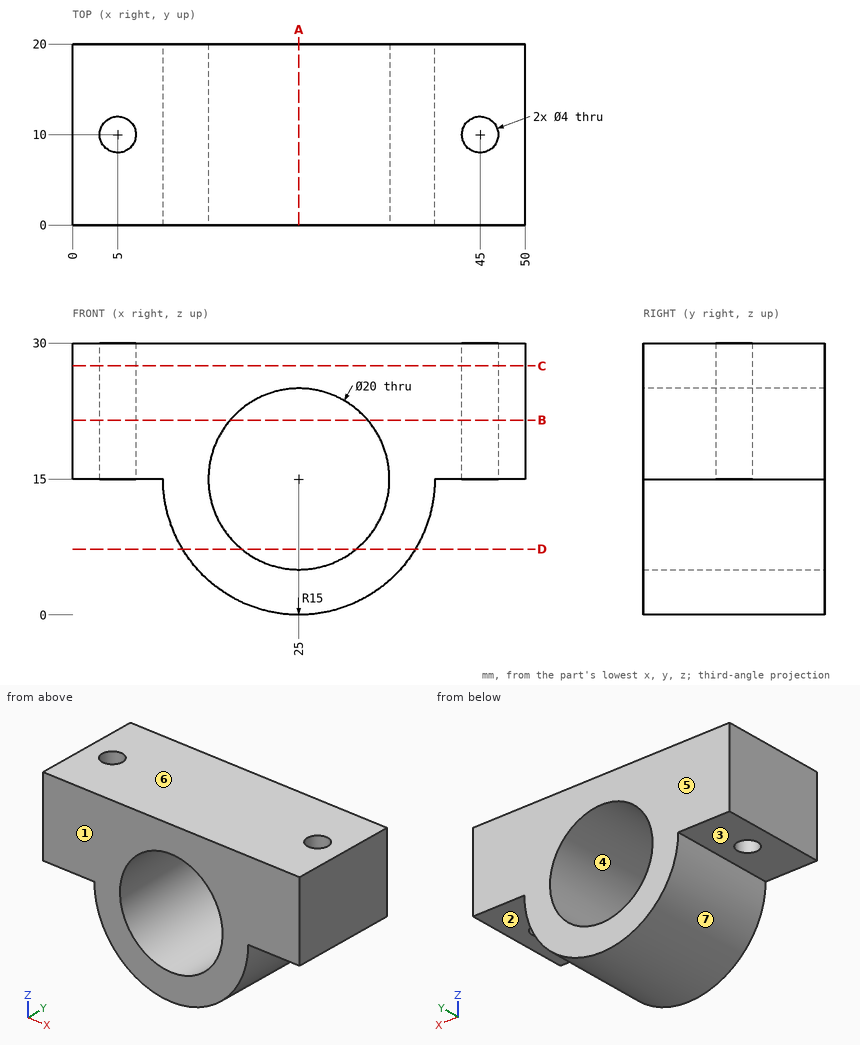
Input: dimensioned drawing with shaded views. Units: mm. Origin: part minimum x, y, z. A direction names the side the tool comes from. Give positions to 0.01 mm unless a question says otherwise; leave off trailing zeros. Order: outer loops, then holes, each group sorted by start corner. A loop starts at its lowest first (then second) coordinate and runs counter-clockwise, first axis right, second up. Notation, with made-up numbers: (22.5, 41.5) -> (33.5, 41.5) arc R19 cw to (33.5, 66.5) -> close; hole circle Ø2 at (-15, 40.25). An arc over 180 degrees is marked (long way). Use a Markdown table: item, result.
1) Section query B-B, the plane z = 21.5. Return the cut outline in (x, y), then the cut area to 3 significant figures.
Answer list:
| item | result |
|---|---|
| outline | (0, 0) -> (17.4, 0) -> (17.4, 20) -> (0, 20) -> close; (32.6, 0) -> (50, 0) -> (50, 20) -> (32.6, 20) -> close; hole circle Ø4 at (5, 10); hole circle Ø4 at (45, 10) |
| area | 671 mm² |
2) Ray query, line 1 along Y through (x, z) = (45, 20); line 2 along Z through (x, y) = (45, 2.5); line 3 along X through (y, z) = (3, 17). Return the intervals inside material, ascending. Write a range as [from, to].
Answer list:
| item | result |
|---|---|
| line 1 | [0, 8], [12, 20] |
| line 2 | [15, 30] |
| line 3 | [0, 15.2], [34.8, 50] |
3) Section query D-D, the plane z = 7.25. Return the cut outline in (x, y).
Answer list:
| item | result |
|---|---|
| outline | (12.16, 0) -> (18.68, 0) -> (18.68, 20) -> (12.16, 20) -> close; (31.32, 0) -> (37.84, 0) -> (37.84, 20) -> (31.32, 20) -> close |
4) Contact query for flat-ended pins moving along their axis: P1, Ø5, axis at x = 45.5, y = 8, coming from the -Z side; P2, Ø12, axis at x = 25.5, z = 17, coming from the -Y side; P3, Ø2, axis at y = 14.5, z = 8, coming from the -X side. Output: stop coordinate, or through.
Answer list:
| item | result |
|---|---|
| P1 | z = 15 |
| P2 | through |
| P3 | x = 11.25 |
5) Section query A-A, the plane x = 25. Return the cut outline in (y, z), then the cut area to 3 significant figures.
Answer list:
| item | result |
|---|---|
| outline | (0, 0) -> (20, 0) -> (20, 5) -> (0, 5) -> close; (0, 25) -> (20, 25) -> (20, 30) -> (0, 30) -> close |
| area | 200 mm² |
6) Reachability of the marked faces 1, 2 and 3 from +Z, -Z, +X, -X, +Y, -Y: full face, straight path, thin tool, end or side. Return the list, or none.
Answer list:
| item | result |
|---|---|
| face 1 | +Z, -Z, +X, -X, -Y |
| face 2 | -Z, +X, +Y, -Y |
| face 3 | -Z, -X, +Y, -Y |
7) Section query C-C, the plane z = 27.5. Return the cut outline in (x, y).
Answer list:
| item | result |
|---|---|
| outline | (0, 0) -> (50, 0) -> (50, 20) -> (0, 20) -> close; hole circle Ø4 at (5, 10); hole circle Ø4 at (45, 10) |
8) Mould query, pull axis Z, two halves, no side actions, for the marked faces 4, 5, 6 and 7. Classes: +Z half, -Z half, draft (parallel to the pull), parting line (faces both ways), or undercut.
Answer list:
| item | result |
|---|---|
| face 4 | undercut |
| face 5 | draft |
| face 6 | +Z half |
| face 7 | -Z half |
